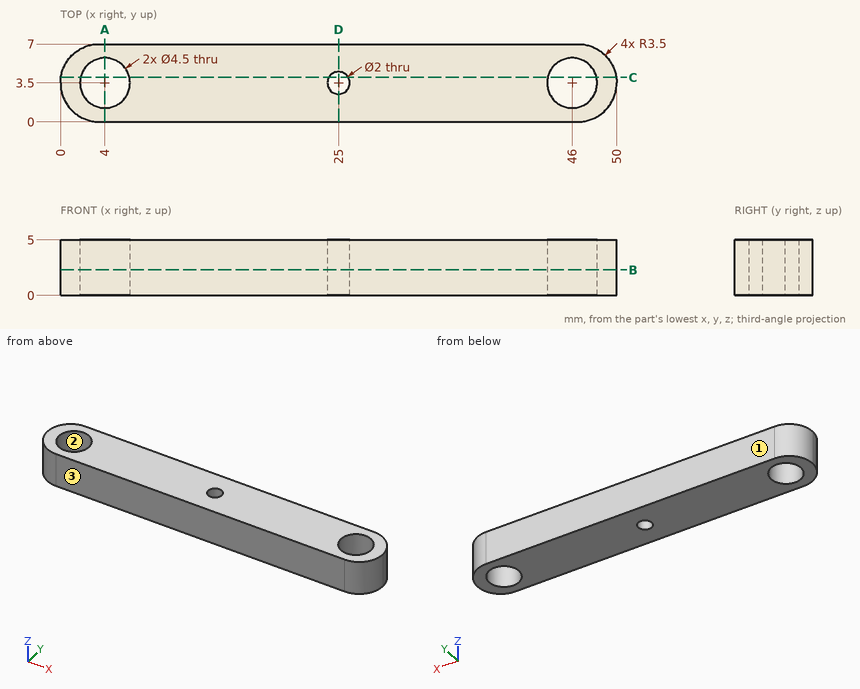
The figure shows three views and two pictorial views of one solid part (mm, origin at its lowest corner). Answer the questions. Round coordinates to 2 decimals unless told otherwise and drop trailing zeros. Loops run counter-clockwise (first coordinate to the right, second up) from the corner with the lowest first, then second, coordinate; pieces in that order, holes last. Notation, with made-up numbers: (48, 58) - (81, 58) arc R22 ccw to (81, 82) - close; hole circle Ø8 at (-20.75, -7). An arc over 180 degrees is marked (long way). One line per question, with ' | ' between items. Start each with the question number.
Q1. Section D-D on x = 25 is taken. Give the vertices of the cut face in (y, z).
Q2. Flat-ended cylindrical pins translate along their axes: pin 1 (1 mm diameter, centred on y = 4.5, z = 3, fed in from -X); pin 2 (3 mm diameter, centred on x = 25, y = 3.5, fed in from +Z). Find the tip coordinate at first contact, or state that the pin passes through.
Q3. For a pull along Y with two mould halves and no side action, classify the marked faces 1, 2 and 3 as +Y half, -Y half, draft (parallel to the pull), parting line (faces both ways), or undercut.
Q4. Section B-B on z = 2.3 is taken. Count the separate pieces of the cut face and the enclosed holes in it, plus the area to 3 significant figures.
Q5. Section A-A on x = 4 is taken. Give the vertices of the cut face in (y, z).
Q6. Find the intervals of material crossed by L1, parallel to Y at x = 4, z = 3.95; L2, parallel to X at y = 4, z = 1.65; L3, parallel to X at y = 3.75, z = 4.05, in increasing order.
Q7. Section C-C on y = 4 is taken. Give the vertices of the cut face in (x, z).
Established:
1) outline: (0, 0) - (2.5, 0) - (2.5, 5) - (0, 5) - close; (4.5, 0) - (7, 0) - (7, 5) - (4.5, 5) - close
2) pin 1: x = 0.04 | pin 2: z = 5
3) face 1: +Y half | face 2: undercut | face 3: -Y half
4) separate pieces: 1 | enclosed holes: 3 | area: 305 mm²
5) outline: (0, 0) - (1.25, 0) - (1.25, 5) - (0, 5) - close; (5.75, 0) - (7, 0) - (7, 5) - (5.75, 5) - close
6) L1: 0 to 1.25, 5.75 to 7 | L2: 0.04 to 1.81, 6.19 to 24.13, 25.87 to 43.81, 48.19 to 49.96 | L3: 0.01 to 1.76, 6.24 to 24.03, 25.97 to 43.76, 48.24 to 49.99
7) outline: (0.04, 0) - (1.81, 0) - (1.81, 5) - (0.04, 5) - close; (6.19, 0) - (24.13, 0) - (24.13, 5) - (6.19, 5) - close; (25.87, 0) - (43.81, 0) - (43.81, 5) - (25.87, 5) - close; (48.19, 0) - (49.96, 0) - (49.96, 5) - (48.19, 5) - close
